from build123d import *

# Parameters (mm, degrees)
SKETCH_13_W               = 25
SKETCH_13_H               = 54
EXTRUDE_6_DEPTH           = 3
EXTRUDE_6_DEPTH_BACK      = 5
SKETCH_16_W               = 22
SKETCH_16_H               = 50
CUT_EXTRUDE_9_DEPTH       = 25
SKETCH_17_W               = 5
SKETCH_17_H               = 15
CUT_EXTRUDE_10_DEPTH      = 30
SKETCH_23_R               = 1.3
CUT_EXTRUDE_11_DEPTH      = 30
CUT_EXTRUDE_11_DEPTH_BACK = 1


with BuildPart() as part:
    # Sketch 13 → Extrude 6 (new body, two sides)
    with BuildSketch(Plane(origin=(95, 0, 0), x_dir=(0, 0, -1), z_dir=(1, 0, 0))) as extrude_6_sk:
        with Locations((112.5, -3)):
            Rectangle(SKETCH_13_W, SKETCH_13_H)
    extrude(amount=EXTRUDE_6_DEPTH)
    extrude(extrude_6_sk.sketch, amount=-EXTRUDE_6_DEPTH_BACK)

    # Sketch 16 → Cut-Extrude 9 (cut)
    with BuildSketch(Plane(origin=(69, 0, 0), x_dir=(0, 0, -1), z_dir=(1, 0, 0))):
        with Locations((111, -3)):
            Rectangle(SKETCH_16_W, SKETCH_16_H)
    extrude(amount=CUT_EXTRUDE_9_DEPTH, mode=Mode.SUBTRACT)

    # Sketch 17 → Cut-Extrude 10 (cut, through all)
    with BuildSketch(Plane(origin=(69, 0, 0), x_dir=(0, 0, -1), z_dir=(1, 0, 0))):
        with Locations((102.5, -3)):
            Rectangle(SKETCH_17_W, SKETCH_17_H)
    extrude(amount=CUT_EXTRUDE_10_DEPTH, mode=Mode.SUBTRACT)

    # Sketch 23 → Cut-Extrude 11 (cut, two sides)
    with BuildSketch(Plane(origin=(69, 0, 0), x_dir=(0, 0, -1), z_dir=(1, 0, 0))) as cut_extrude_11_sk:
        with Locations((119.7, 16.7)):
            Circle(SKETCH_23_R)
        with Locations((103.3, -24.2)):
            Circle(SKETCH_23_R)
    extrude(amount=CUT_EXTRUDE_11_DEPTH, mode=Mode.SUBTRACT)
    extrude(cut_extrude_11_sk.sketch, amount=-CUT_EXTRUDE_11_DEPTH_BACK, mode=Mode.SUBTRACT)


solid = part.part
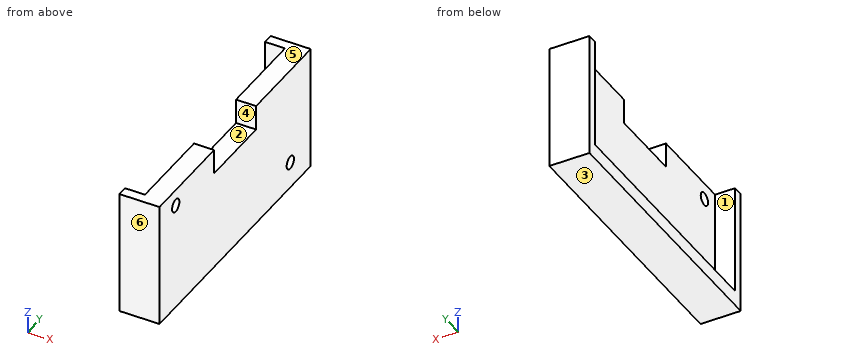
Work out the finished part from the listing and answer in its coordinate system (mm). Face numbers are marked on the shaded views. A direction names the side the tool comes from. Round coordinates to 2 decimals unless told otherwise and drop trailing zeros. Write each loop counter-clockwise with the first axis right and the second up, starting at its lowest first coordinate (ties: lowest second). Pieces come first, ordered by that corner, then holes. Notation, with made-up numbers: (20, 14.25) - (31, 14.25) arc R26 cw to (31, 49.25) - close; hole circle Ø2 at (-34, 23.25). An arc over 180 degrees is marked (long way). Answer in a Markdown table with one row per item. Add a question column.
1. For the marked faces 1, 2 and 3, determine the directions among +Z, -Z, +X, -X, +Y, -Y from which every point of the face is accessible in a straight line to the end or side of a thin tool.
2. Find the intervals of material crossed by line 1 along Y through (x, z) = (96, -103.3); line 2 along Z through (x, y) = (95.65, -24.2); line 3 along Y through (x, z) = (91, -116.75), in increasing order. Write a range as from..to.
3. A cutting plane is placed at A-A, the plane z = -119.7. Determine the outline of the cut face in (x, y).
4. The mould has two halves that part along Y. Classify the marked faces 4, 5 and 6: +Y half, -Y half, draft (parallel to the pull), parting line (faces both ways), or undercut.
5. Given pin 1 (1.5 mm diameter, centred on y = 17.5, z = -103.5, fed in from -X); pin 2 (3 mm diameter, centred on x = 96, y = -3, fed in from +Z); pin 3 (6 mm diameter, centred on y = -6.5, z = -120.5, fed in from -X); pin 4 (3 mm diameter, centred on x = 92, y = -10, fed in from +Z), each flat-ended and moving along its own axis, determine where each tip first touches the part or whether it passes through.
6. A cutting plane is placed at C-C, the plane z = -103.3. Determine the outline of the cut face in (x, y).
7. A cutting plane is placed at B-B, the plane y = 16.7. Determine the outline of the cut face in (x, z).
8. A cutting plane is placed at D-D, the plane x = 95.75. Determine the outline of the cut face in (y, z).
Worked out:
| question | item | result |
|---|---|---|
| 1 | face 1 | +Z, -X |
| 1 | face 2 | +Z, +X, -X |
| 1 | face 3 | -Z, +X, -X, +Y, -Y |
| 2 | line 1 | -30..-25.5, -22.9..-10.5, 4.5..24 |
| 2 | line 2 | -125..-104.6, -102..-100 |
| 2 | line 3 | -30..-28, 22..24 |
| 3 | outline | (90, -30) - (98, -30) - (98, 15.4) - (94, 15.4) - (94, -28) - (90, -28) - close; (90, 22) - (94, 22) - (94, 18) - (98, 18) - (98, 24) - (90, 24) - close |
| 4 | face 4 | undercut |
| 4 | face 5 | draft |
| 4 | face 6 | -Y half |
| 5 | pin 1 | x = 94 |
| 5 | pin 2 | z = -105 |
| 5 | pin 3 | x = 90 |
| 5 | pin 4 | z = -122 |
| 6 | outline | (90, -30) - (98, -30) - (98, -25.5) - (94, -25.5) - (94, -28) - (90, -28) - close; (90, 22) - (94, 22) - (94, 4.5) - (98, 4.5) - (98, 24) - (90, 24) - close; (94, -22.9) - (98, -22.9) - (98, -10.5) - (94, -10.5) - close |
| 7 | outline | (90, -125) - (98, -125) - (98, -121) - (94, -121) - (94, -122) - (90, -122) - close; (94, -118.4) - (98, -118.4) - (98, -100) - (94, -100) - close |
| 8 | outline | (-30, -125) - (24, -125) - (24, -100) - (4.5, -100) - (4.5, -105) - (-10.5, -105) - (-10.5, -100) - (-30, -100) - close; hole circle Ø2.6 at (-24.2, -103.3); hole circle Ø2.6 at (16.7, -119.7) |
